Autodesk Inventor part; units mm, degrees
ref_plane "YZ Plane" through (0, 0, 0) normal (1, 0, 0) x (0, 1, 0)
ref_plane "XZ Plane" through (0, 0, 0) normal (0, 1, 0) x (-1, 0, 0)
ref_plane "XY Plane" through (0, 0, 0) normal (0, 0, 1) x (1, 0, 0)
sketch "スケッチ2" plane through (0, 0, 0) normal (1, 0, 0) x (0, 1, 0)
  line L0 (0, 0) -> (-84.4498, 0)
  line L1 (-84.4498, -20) -> (1.7498, -20)
  line L2 (0, 0) -> (83.1668, 14.6646)
  line L3 (86.6398, -5.0316) -> (1.7498, -20)
  arc A0 (87.251, 14.537) -> (83.1668, 14.6646) centre (84.9033, 4.8165) ccw
  arc A1 (86.6398, -5.0316) -> (90.434, -3.5148) centre (84.9033, 4.8165) ccw
  arc A2 (-88.4498, -19.1652) -> (-84.4498, -20) centre (-84.4498, -10) ccw
  arc A3 (-84.4498, 0) -> (-88.4498, -0.8348) centre (-84.4498, -10) ccw
  arc A4 (-84.4498, -14) -> (-84.4498, -6) centre (-84.4498, -10) ccw
  line L4 (-84.4498, -6) -> (-88.4498, -6)
  line L5 (-84.4498, -14) -> (-88.4498, -14)
  line L6 (-88.4498, -0.8348) -> (-88.4498, -6)
  line L7 (-88.4498, -14) -> (-88.4498, -19.1652)
  line L8 (87.251, 14.537) -> (88.1479, 9.4503)
  line L9 (89.5371, 1.5718) -> (90.434, -3.5148)
  line L10 (1.7498, -20) -> (0, 0)
  line L11 (88.1479, 9.4503) -> (89.5371, 1.5718)
  dimension "d21" = 20
  dimension "d22" = 10
  dimension "d23" = 170
  dimension "d27" = 10
  dimension "d31" = 8
  dimension "d33" = 4
  dimension "d35" = 4
  dimension "d36" = 170
  dimension "d139" = 20
extrude "押し出し1" add sketch "スケッチ2" along normal blind 2
sketch "スケッチ4" plane through (0, 0, 0) normal (-1, 0, 0) x (0, 0, 1)
  line L0 (-20, 1.7498) -> (-5.0316, 86.6398)
  line L1 (-20, -84.4498) -> (-20, 1.7498)
  circle A0 centre (-17, -18.5891) radius 1
  circle A1 centre (-13.5138, 21.2587) radius 1
  line L2 (-17, -18.5891) -> (-13.5138, 21.2587)
  line L3 (-20, 1.7498) -> (0, 0)
  dimension "d57" = 2
  dimension "d59" = 40
  dimension "d60" = 175
  dimension "d61" = 3
  dimension "d62" = 3
hole "穴2" at (0, -18.5891, -17) at (0, 21.2587, -13.5138) direction (1, 0, 0) diameter 1.6 end through all
sketch "スケッチ6" plane through (2, 0, 0) normal (1, 0, 0) x (0, 0, -1)
  line L0 (20, 1.7498) -> (5.0316, 86.6398)
  arc A0 (5.0316, 86.6398) -> (3.5148, 90.434) centre (-4.8165, 84.9033) ccw
  line L1 (3.5148, 90.434) -> (-14.537, 87.251)
  arc A1 (-14.537, 87.251) -> (-14.6646, 83.1668) centre (-4.8165, 84.9033) ccw
  line L2 (-14.6646, 83.1668) -> (0, 0)
  line L3 (-9.3978, 53.2975) -> (-12.6117, 57.1277)
  line L4 (-14.537, 87.251) -> (-17.8212, 86.6719)
  line L5 (-17.8212, 86.6719) -> (-12.6117, 57.1277)
  line L6 (3.5148, 90.434) -> (6.799, 91.0131)
  line L7 (6.799, 91.0131) -> (12.0085, 61.4689)
  line L8 (12.0085, 61.4689) -> (10.2984, 56.7704)
  dimension "d75" = 150
  dimension "d76" = 150
  dimension "d77" = 2.5
  dimension "d78" = 2.5
  dimension "d79" = 30
extrude "押し出し2" [suppressed]
sketch "スケッチ5" plane through (2, 0, 0) normal (1, 0, 0) x (0, 0, -1)
  line L0 (3.5148, 90.434) -> (-14.537, 87.251)
  circle A0 centre (-12.5213, 82.5293) radius 1.5
  circle A1 centre (3.2356, 85.3077) radius 1.5
  line L1 (5.0316, 86.6398) -> (20, 1.7498)
  line L2 (20, 1.7498) -> (20, -84.4498)
  arc A2 (19.1652, -88.4498) -> (20, -84.4498) centre (10, -84.4498) ccw
  line L3 (19.1652, -88.4498) -> (14, -88.4498)
  line L4 (14, -88.4498) -> (14, -84.4498)
  arc A3 (14, -84.4498) -> (6, -84.4498) centre (10, -84.4498) ccw
  line L5 (6, -84.4498) -> (6, -88.4498)
  line L6 (6, -88.4498) -> (0.8348, -88.4498)
  arc A4 (0, -84.4498) -> (0.8348, -88.4498) centre (10, -84.4498) ccw
  line L7 (0, -84.4498) -> (0, 0)
  line L8 (0, 0) -> (-14.6646, 83.1668)
  circle A5 centre (17, -18.5891) radius 0.8
  circle A6 centre (13.5138, 21.2587) radius 0.8
  arc A7 (-14.537, 87.251) -> (-14.6646, 83.1668) centre (-4.8165, 84.9033) ccw
  line L9 (-14.537, 87.251) -> (3.5148, 90.434)
  arc A8 (5.0316, 86.6398) -> (3.5148, 90.434) centre (-4.8165, 84.9033) ccw
  dimension "d70" = 5
  dimension "d71" = 5
  dimension "d72" = 3
  dimension "d114" = 16
hole "穴3" [suppressed]
sketch "スケッチ7" plane through (2, 0, 0) normal (1, 0, 0) x (0, 0, -1)
  arc A0 (0, -84.4498) -> (0.8348, -88.4498) centre (10, -84.4498) ccw
  line L0 (0.8348, -88.4498) -> (6, -88.4498)
  circle A1 centre (3, -84.4498) radius 1
  dimension "d89" = 4
  dimension "d90" = 7
  dimension "d91" = 2
hole "穴4" at (2, -84.4498, -3) direction (-1, 0, 0) diameter 2 end through all
pattern_circular "円形状パターン3" count 5 over 180 about axis through (0, -84.4498, -10) along (-1, 0, 0) of "穴4"
sketch "スケッチ8" plane through (2, 0, 0) normal (1, 0, 0) x (0, 0, -1)
  line L0 (3.5148, 90.434) -> (-14.537, 87.251)
  line L1 (-17.8212, 86.6719) -> (-12.6117, 57.1277)
  circle A0 centre (-11.4794, 76.6205) radius 1.5
  circle A1 centre (4.2775, 79.3988) radius 1.5
  point P0 (6.799, 91.0131)
  dimension "d102" = 11
  dimension "d103" = 11
  dimension "d104" = 16
  dimension "d105" = 4.5
  dimension "d106" = 3
hole "穴5" [suppressed]
sketch "スケッチ11" plane through (2, 0, 0) normal (1, 0, 0) x (0, 0, -1)
  circle A0 centre (-11.4794, 76.6205) radius 1.75
  circle A1 centre (4.2775, 79.3988) radius 1.75
  line L0 (-17.8212, 86.6719) -> (-12.6117, 57.1277)
  circle A2 centre (-8.8747, 61.8483) radius 1.5
  circle A3 centre (6.8822, 64.6267) radius 1.5
  dimension "d124" = 3
  dimension "d126" = 16
  dimension "d127" = 15
  dimension "d128" = 4.5
  dimension "d130" = 15
hole "穴6" [suppressed]
sketch "スケッチ13" plane through (2, 0, 0) normal (1, 0, 0) x (0, 0, -1)
  line L0 (0, 0) -> (0, -84.4498)
  line L1 (20, -84.4498) -> (20, 1.7498)
  line L2 (20, 1.7498) -> (5.0316, 86.6398)
  line L3 (3.5148, 90.434) -> (-14.537, 87.251)
  line L4 (-14.6646, 83.1668) -> (0, 0)
  line L5 (-3.8662, 44.9615) -> (9.2538, 39.6592)
  line L6 (9.2538, 39.6592) -> (6.6491, 54.4313)
  line L7 (6.6491, 54.4313) -> (-3.8662, 44.9615)
  line L8 (-2.1297, 35.1134) -> (10.9903, 29.8111)
  line L9 (10.9903, 29.8111) -> (0.475, 20.3413)
  line L10 (0.475, 20.3413) -> (-2.1297, 35.1134)
  line L11 (2.7324, 7.5388) -> (13.2477, 17.0086)
  line L12 (13.2477, 17.0086) -> (15.8525, 2.2365)
  line L13 (15.8525, 2.2365) -> (2.7324, 7.5388)
  line L14 (4, -2.2635) -> (16, -9.7635)
  line L15 (4, -17.2635) -> (4, -2.2635)
  line L16 (16, -9.7635) -> (4, -17.2635)
  line L17 (4, -30.2635) -> (16, -22.7635)
  line L18 (16, -22.7635) -> (16, -37.7635)
  line L19 (16, -37.7635) -> (4, -30.2635)
  line L20 (4, -55.2635) -> (16, -47.7635)
  line L21 (16, -47.7635) -> (4, -40.2635)
  line L22 (4, -40.2635) -> (4, -55.2635)
  line L23 (4, -65.2635) -> (16, -57.7635)
  line L24 (16, -57.7635) -> (16, -72.7635)
  line L25 (16, -72.7635) -> (4, -65.2635)
  point P0 (10.2984, 56.7704)
  point P1 (6.799, 91.0131)
  point P2 (-17.8212, 86.6719)
  point P3 (-9.3978, 53.2975)
  dimension "d141" = 15
  dimension "d144" = 4
  dimension "d145" = 36
  dimension "d146" = 12
  dimension "d147" = 4
  dimension "d149" = 4
  dimension "d160" = 4
  dimension "d162" = 61
  dimension "d163" = 74
  dimension "d164" = 12
  dimension "d165" = 13
  dimension "d166" = 4
  dimension "d167" = 4
  dimension "d168" = 10
  dimension "d169" = 4
  dimension "d170" = 10
extrude "押し出し4" [suppressed]
fillet "フィレット1" [suppressed]
sketch "スケッチ14" plane through (2, 0, 0) normal (1, 0, 0) x (0, 0, -1)
  line L0 (3.5148, 90.434) -> (-14.537, 87.251)
  arc A0 (-14.537, 87.251) -> (-14.6646, 83.1668) centre (-4.8165, 84.9033) ccw
  arc A1 (-8.7557, 84.2087) -> (-0.8772, 85.5979) centre (-4.8165, 84.9033) ccw
  line L1 (-8.7557, 84.2087) -> (-9.4503, 88.1479)
  line L2 (-0.8772, 85.5979) -> (-1.5718, 89.5371)
  dimension "d174" = 8
extrude "押し出し5" cut sketch "スケッチ14" against normal blind 2
sketch "スケッチ15" plane through (2, 0, 0) normal (1, 0, 0) x (0, 0, -1)
  line L0 (-9.4503, 88.1479) -> (-14.537, 87.251)
  arc A0 (-14.537, 87.251) -> (-14.6646, 83.1668) centre (-4.8165, 84.9033) ccw
  circle A1 centre (-11.7101, 83.6878) radius 1
  dimension "d178" = 2
  dimension "d180" = 4
  dimension "d181" = 7
hole "穴7" at (2, 83.6878, 11.7101) direction (-1, 0, 0) diameter 2 end through all
pattern_circular "円形状パターン4" count 5 over 180 about axis through (2, 84.9033, 4.8165) along (1, 0, 0) of "穴7"
properties part number "Arm_Link_1" material "アルミニウム 6061"
Geometry check sheet. Reference: the model listing, model coordinates, mm. Give positions to 0.01 mm unless a question says otherwise; leave off trailing zeros. Loops run counter-clockwise (first coordinate to the right, second up) from the corner with the lowest first, then second, coordinate; pieces in that order, holes last. Notation, with made-up numbers: M 77.5,-37 L 127.5,-37 A20 ccw 127.5,-2 Z; hole C 8.5,44.5 d10. An arc over 180 degrees is marked long. Write item = value, one per line. Start each with the question number.
1. Section check B-B, the plane y = 32.5. Enter the section's corners in (x, z).
2. Draft check along Z on faces 1 (the face through (1.01, 80.95, 4.21)), 2 (the face through (2, 0, -6)), 3 (the face through (0.99, 44.79, -12.41)). Enter one of: +Z half, -Z half, draft (parallel to the pull), parting line (faces both ways), or undercut.
3. Thickness scan on probe 1 along Z at (x, y) = (1.7, -29); probe 2 along Z at (x, y) = (1.6, 50.5). Record the ranges inside material, lowest first.
4. Section check A-A, the plane y = -66. Enter the section's corners in (x, z), plus the area to 3 significant figures.
5. Go/stop test with flat-tipped pins: P1, Ø0.6, axis at x = 1.5, y = -86, coming from the -Z side; P2, Ø0.6, axis at x = 1, y = -37, coming from the +Z side. Record where each tip stops, or that it passes through.
Values follow:
q1.outline = M 0,-14.58 L 2,-14.58 L 2,5.73 L 0,5.73 Z
q2.face_1 = undercut
q2.face_2 = draft
q2.face_3 = -Z half
q3.probe_1 = -20 to 0
q3.probe_2 = -11.4 to 8.9
q4.outline = M 0,-20 L 2,-20 L 2,0 L 0,0 Z
q4.area = 40.0 mm^2
q5.P1 = -19.92
q5.P2 = 0
